Autodesk Inventor part; units mm, degrees
ref_plane "YZ Plane" through (0, 0, 0) normal (1, 0, 0) x (0, 1, 0)
ref_plane "XZ Plane" through (0, 0, 0) normal (0, 1, 0) x (-1, 0, 0)
ref_plane "XY Plane" through (0, 0, 0) normal (0, 0, 1) x (1, 0, 0)
sketch "Sketch1" plane through (0, 0, 0) normal (0, 1, 0) x (-1, 0, 0)
  line L0 (50, 75) -> (-50, 75)
  line L1 (-50, -75) -> (50, -75)
  line L2 (50, 50) -> (43.65, 50)
  line L3 (43.65, 50) -> (43.65, -50)
  line L4 (43.65, -50) -> (50, -50)
  line L5 (-50, 50) -> (-43.65, 50)
  line L6 (-43.65, 50) -> (-43.65, -50)
  line L7 (-43.65, -50) -> (-50, -50)
  line L8 (50, -75) -> (50, -50)
  line L9 (50, 50) -> (50, 75)
  line L10 (-50, 75) -> (-50, 50)
  line L11 (-50, -50) -> (-50, -75)
  line L12 (28.65, 50) -> (-28.65, 50)
  line L13 (-28.65, 50) -> (-28.65, -50)
  line L14 (-28.65, -50) -> (28.65, -50)
  line L15 (28.65, -50) -> (28.65, 50)
  point P0 (0, 0)
  point P1 (50, 0)
  point P2 (0, -75)
  point P3 (43.65, 0)
  point P4 (28.65, 0)
  point P5 (0, -50)
  point P6 (0, 50)
  point P7 (46.825, 50)
  dimension "d1" = 150
  dimension "d5" = 25
  dimension "d6" = 25
  dimension "d7" = 6.35
  dimension "d8" = 6.35
  dimension "d9" = 100
  dimension "d10" = 100
  dimension "d11" = 6.35
  dimension "d12" = 15
extrude "Extrusion1" add sketch "Sketch1" along normal blind 6.35
properties part number "TopHolderV1"
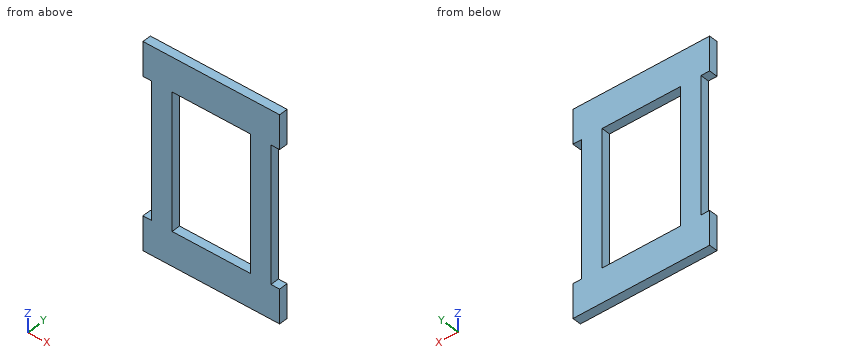
Source: CAD feature listing. Evaluate the final solid. Frame: model axes, mm. Give positions to 0.01 mm unless a question says otherwise; leave off trailing zeros. Write each loop counter-clockwise with the first axis right and the second up, starting at its lowest first coordinate (ties: lowest second). Pieces come first, ordered by that corner, then holes. Notation, with made-up numbers: M 3,4 L 28,4 A15 cw 28,18 Z; hole C 4,-15.75 d9. An arc over 180 degrees is marked long. Answer as a JSON object with one key per item and string values.
Q1. Ray query, line 1 along Z through (x, y) = (2.5, 4.25); line 2 along X through (y, z) = (3.25, 45.5). Return the intervals inside material, ascending.
Geometry check:
{"line 1": "z = -75 to -50, 50 to 75", "line 2": "x = -43.65 to -28.65, 28.65 to 43.65"}
Q2. Cut plane C-C, the plane y = 2. Return the cut outline in (x, z), then the cut area to 3 significant figures.
Geometry check:
{"outline": "M -50,-75 L 50,-75 L 50,-50 L 43.65,-50 L 43.65,50 L 50,50 L 50,75 L -50,75 L -50,50 L -43.65,50 L -43.65,-50 L -50,-50 Z; hole M -28.65,-50 L 28.65,-50 L 28.65,50 L -28.65,50 Z", "area": "8,000 mm^2"}
Q3. Cut plane A-A, the plane x = -27. Return the cut outline in (y, z).
Geometry check:
{"outline": "M 0,-75 L 6.35,-75 L 6.35,-50 L 0,-50 Z; M 0,50 L 6.35,50 L 6.35,75 L 0,75 Z"}
Q4. Cut plane B-B, the plane z = -39. Return the cut outline in (x, y), then the cut area to 4 significant figures.
Geometry check:
{"outline": "M -43.65,0 L -28.65,0 L -28.65,6.35 L -43.65,6.35 Z; M 28.65,0 L 43.65,0 L 43.65,6.35 L 28.65,6.35 Z", "area": "190.5 mm^2"}
Q5. Contact query for flat-ended pins moving along their axis: P1, Ø1.9, axis at y = 3, z = -18.5, coming from the -X side; P2, Ø4, axis at x = -34.5, z = 4, coming from the -Y side. Output: stop coordinate, or through.
Geometry check:
{"P1": "stops at x = -43.65", "P2": "stops at y = 0"}
